from build123d import *

# Parameters (mm, degrees)
SKETCH1_W            = 40
SKETCH1_H            = 50
BOSS_EXTRUDE1_DEPTH  = 5
SKETCH3_W            = 5
SKETCH3_H            = 5
BOSS_EXTRUDE5_DEPTH  = 20
SKETCH3_3_W          = 15
SKETCH3_3_H          = 5
SKETCH3_3_W_2        = 5
BOSS_EXTRUDE6_DEPTH  = 10
CUT_EXTRUDE3_DEPTH   = 4
BOSS_EXTRUDE9_START  = 3
BOSS_EXTRUDE9_DEPTH  = 3
SKETCH11_W           = 5
SKETCH11_H           = 5
BOSS_EXTRUDE10_DEPTH = 5
SKETCH12_R           = 1.5
CUT_EXTRUDE4_DEPTH   = 5
SKETCH14_W           = 5
SKETCH14_H           = 5
SKETCH14_W_2         = 10
BOSS_EXTRUDE12_DEPTH = 30
SKETCH15_W           = 40
SKETCH15_H           = 15
BOSS_EXTRUDE13_DEPTH = 5
BOSS_EXTRUDE15_DEPTH = 15
BOSS_EXTRUDE17_DEPTH = 10
SKETCH18_W           = 5
SKETCH18_H           = 15
BOSS_EXTRUDE18_DEPTH = 40
BOSS_EXTRUDE19_DEPTH = 9
SKETCH20_W           = 5
SKETCH20_H           = 5
BOSS_EXTRUDE20_DEPTH = 5
SKETCH21_R           = 1.5
CUT_EXTRUDE5_DEPTH   = 5
SKETCH22_W           = 5
SKETCH22_H           = 5
BOSS_EXTRUDE21_DEPTH = 5
SKETCH23_R           = 1.5
CUT_EXTRUDE6_DEPTH   = 5
SKETCH24_R           = 1.05
CUT_EXTRUDE7_DEPTH   = 5


with BuildPart() as part:
    # Sketch1 → Boss-Extrude1 (new body)
    with BuildSketch(Plane(origin=(0, 0, 0), x_dir=(1, 0, 0), z_dir=(0, 1, 0))):
        Rectangle(SKETCH1_W, SKETCH1_H)
    extrude(amount=BOSS_EXTRUDE1_DEPTH)

    # Sketch3 → Boss-Extrude5 (add)
    with BuildSketch(Plane(origin=(0, 5, 0), x_dir=(1, 0, 0), z_dir=(0, 1, 0))):
        with Locations((9.5, 22.5)):
            Rectangle(SKETCH3_W, SKETCH3_H)
    extrude(amount=BOSS_EXTRUDE5_DEPTH)

    # Sketch3_3 → Boss-Extrude6 (add)
    with BuildSketch(Plane(origin=(0, 5, 0), x_dir=(1, 0, 0), z_dir=(0, 1, 0))):
        with Locations((-0.5, 22.5)):
            Rectangle(SKETCH3_3_W, SKETCH3_3_H)
        Polygon((-16, -20), (-16, 25), (-20, 25), (-20, -25), (7, -25), (7, -20), align=None)
        with Locations((17.5, -22.5)):
            Rectangle(SKETCH3_3_W_2, SKETCH3_3_H)
    extrude(amount=BOSS_EXTRUDE6_DEPTH)

    # Sketch8 → Cut-Extrude3 (cut)
    with BuildSketch(Plane.ZY.offset(20)):
        with BuildLine():
            Line((1, 15), (-21, 15))
            ThreePointArc((-21, 15), (-10, 4), (1, 15))
        make_face()
    extrude(amount=-CUT_EXTRUDE3_DEPTH, mode=Mode.SUBTRACT)

    # Sketch10 → Boss-Extrude9 (add)
    with BuildSketch(Plane.ZY.offset(20).offset(BOSS_EXTRUDE9_START)):
        with BuildLine():
            Line((1, 15), (4, 15))
            Line((4, 15), (4, 0))
            Line((4, 0), (-24, 0))
            Line((-24, 0), (-24, 15))
            Line((-24, 15), (-21, 15))
            ThreePointArc((-21, 15), (-10, 4), (1, 15))
        make_face()
    extrude(amount=-BOSS_EXTRUDE9_DEPTH)

    # Sketch11 → Boss-Extrude10 (add)
    with BuildSketch(Plane(origin=(0, 0, -25), x_dir=(-1, 0, 0), z_dir=(0, 0, -1))):
        with Locations((0, 12.5)):
            Rectangle(SKETCH11_W, SKETCH11_H)
    extrude(amount=BOSS_EXTRUDE10_DEPTH)

    # Sketch12 → Cut-Extrude4 (cut)
    with BuildSketch(Plane.XZ.offset(-10)):
        with Locations(Location((0, -27.5, 0), (0, 0, 270))):
            Circle(SKETCH12_R)
    extrude(amount=-CUT_EXTRUDE4_DEPTH, mode=Mode.SUBTRACT)

    # Sketch14 → Boss-Extrude12 (add)
    with BuildSketch(Plane.XY.offset(25)):
        with Locations((17.5, 12.5)):
            Rectangle(SKETCH14_W, SKETCH14_H)
        with Locations((-17.5, 12.5)):
            Rectangle(SKETCH14_W, SKETCH14_H)
        with Locations((0, 2.5)):
            Rectangle(SKETCH14_W_2, SKETCH14_H)
    extrude(amount=BOSS_EXTRUDE12_DEPTH)

    # Sketch15 → Boss-Extrude13 (add)
    with BuildSketch(Plane.XY.offset(55)):
        with Locations((0, 7.5)):
            Rectangle(SKETCH15_W, SKETCH15_H)
    extrude(amount=BOSS_EXTRUDE13_DEPTH)

    # Sketch16 → Boss-Extrude15 (add)
    with BuildSketch(Plane(origin=(20, 0, 0), x_dir=(0, 0, -1), z_dir=(1, 0, 0))):
        Polygon((-60, 0), (-55, 0), (-55, 10), (-55, 15), (-60, 15), align=None)
    extrude(amount=BOSS_EXTRUDE15_DEPTH)

    # Sketch17 → Boss-Extrude17 (add)
    with BuildSketch(Plane.ZY.offset(20)):
        Polygon((55, 0), (60, 0), (60, 15), (55, 15), (55, 10), align=None)
    extrude(amount=BOSS_EXTRUDE17_DEPTH)

    # Sketch18 → Boss-Extrude18 (add)
    with BuildSketch(Plane.XY.offset(60)):
        with Locations((32.5, 7.5)):
            Rectangle(SKETCH18_W, SKETCH18_H)
        with Locations((-27.5, 7.5)):
            Rectangle(SKETCH18_W, SKETCH18_H)
    extrude(amount=BOSS_EXTRUDE18_DEPTH)

    # Sketch19 → Boss-Extrude19 (add)
    with BuildSketch(Plane(origin=(-25, 0, 0), x_dir=(0, 0, -1), z_dir=(1, 0, 0))):
        with BuildLine():
            Line((-86, 15), (-94, 15))
            ThreePointArc((-94, 15), (-90, 11), (-86, 15))
        make_face()
    extrude(amount=BOSS_EXTRUDE19_DEPTH)

    # Sketch20 → Boss-Extrude20 (add)
    with BuildSketch(Plane.ZY.offset(30)):
        with Locations((87.5, 12.5)):
            Rectangle(SKETCH20_W, SKETCH20_H)
    extrude(amount=BOSS_EXTRUDE20_DEPTH)

    # Sketch21 → Cut-Extrude5 (cut)
    with BuildSketch(Plane.XZ.offset(-10)):
        with Locations(Location((-32.5, 87.5, 0), (0, 0, 270))):
            Circle(SKETCH21_R)
    extrude(amount=-CUT_EXTRUDE5_DEPTH, mode=Mode.SUBTRACT)

    # Sketch22 → Boss-Extrude21 (add)
    with BuildSketch(Plane(origin=(35, 0, 0), x_dir=(0, 0, -1), z_dir=(1, 0, 0))):
        with Locations((-87.5, 12.5)):
            Rectangle(SKETCH22_W, SKETCH22_H)
    extrude(amount=BOSS_EXTRUDE21_DEPTH)

    # Sketch23 → Cut-Extrude6 (cut)
    with BuildSketch(Plane.XZ.offset(-10)):
        with Locations(Location((37.5, 87.5, 0), (0, 0, 270))):
            Circle(SKETCH23_R)
    extrude(amount=-CUT_EXTRUDE6_DEPTH, mode=Mode.SUBTRACT)

    # Sketch24 → Cut-Extrude7 (cut)
    with BuildSketch(Plane.ZY.offset(-30)):
        with Locations((93.5, 11.5)):
            Circle(SKETCH24_R)
        with Locations((86.5, 11.5)):
            Circle(SKETCH24_R)
    extrude(amount=-CUT_EXTRUDE7_DEPTH, mode=Mode.SUBTRACT)


solid = part.part
For this review, take the finished solid that the model builds, in its own axes (mm). A direction names the side the tool comes from. Coordinates: 2 decimals unless noted, no trailing zeros. Loops run counter-clockwise (first coordinate to the right, second up) from the corner with the lowest first, then second, coordinate; pieces in that order, holes last. Notation, with made-up numbers: (49, 65.25) - (102, 65.25) arc R20 ccw to (102, 104.25) - close; hole circle Ø6 at (80.25, 88). An arc over 180 degrees is marked (long way). Use a Markdown table: item, result. Add a question column.
Item 1: Insertion check: pin 1 Ø3 at (x, y) = (-10, 9) entering from -Z; pin 2 Ø8 at (x, z) = (15.5, 45) entering from -Y; pin 3 Ø6 at (x, z) = (9, 29.5) entering from +Y; pin 4 Ø12 at (x, y) = (28, 7) entering from +Z. Each pin has a flat end and moves straight along its axis. Give the tip position at first contact, or say it passes through.
Item 2: We need section B-B (x = -32.5). Give the boundary of the cut face in (y, z), and give its area (3 significant figures).
Item 3: Tool access review of faces 1 (the face through (39, 10, 89)), 2 (the face through (-4, 10, 20)), 3 (the face through (12, 15, -22)): name each direction out of +Z, -Z, +X, -X, +Y, -Y from which nothing blocks a thin tool from reaching the whole face with its end or side.
Item 4: We need section D-D (y = 21.75). Give the boundary of the cut face in (x, z).
Item 5: We need section A-A (z = 46.5). Give the boundary of the cut face in (x, y), and give its area (3 significant figures).
Item 6: For line 1 (X direction, y = 4.5, z = 82); line 2 (X direction, y = 11.65, z = 87.5); line 3 (Z direction, x = 8, y = 6), list the stretches that pass through material, from the lowest coordinate up.
Item 7: Mouldability with a two-part tool opening along X and no side actions: class faces 4 (the face through (-8, 10, -22)), 5 (the face through (-16, 13, 90)), 6 (the face through (-1, 15, -23)), 7 (the face through (-2.5, 12, -27)) as pulls with the +X half, pulls with the -X half, needs draft (parallel to the pull), parting line crosses it, or undercut.
Item 8: We need section C-C (z = -27.5). Give the boundary of the cut face in (x, y), and give its area (3 significant figures).
Results list:
| question | item | result |
|---|---|---|
| 1 | pin 1 | stops at z = 20 |
| 1 | pin 2 | stops at y = 10 |
| 1 | pin 3 | passes through |
| 1 | pin 4 | stops at z = 100 |
| 2 | outline | (10, 85) - (15, 85) - (15, 86) - (10, 86) - close; (10, 89) - (15, 89) - (15, 90) - (10, 90) - close |
| 2 | area | 10.0 mm^2 |
| 3 | face 1 | +Z, -Z, +X, -Y |
| 3 | face 2 | +X, +Y |
| 3 | face 3 | -Z, +X, +Y |
| 4 | outline | (7, -25) - (12, -25) - (12, -20) - (7, -20) - close |
| 5 | outline | (-20, 10) - (-15, 10) - (-15, 15) - (-20, 15) - close; (-5, 0) - (5, 0) - (5, 5) - (-5, 5) - close; (15, 10) - (20, 10) - (20, 15) - (15, 15) - close |
| 5 | area | 100 mm^2 |
| 6 | line 1 | x = -30 to -25, 30 to 35 |
| 6 | line 2 | x = -35 to -34, -31 to -25, 35 to 36, 39 to 40 |
| 6 | line 3 | z = -25 to -20, 55 to 60 |
| 7 | face 4 | undercut |
| 7 | face 5 | undercut |
| 7 | face 6 | needs draft |
| 7 | face 7 | pulls with the -X half |
| 8 | outline | (-2.5, 10) - (-1.5, 10) - (-1.5, 15) - (-2.5, 15) - close; (1.5, 10) - (2.5, 10) - (2.5, 15) - (1.5, 15) - close |
| 8 | area | 10.0 mm^2 |
